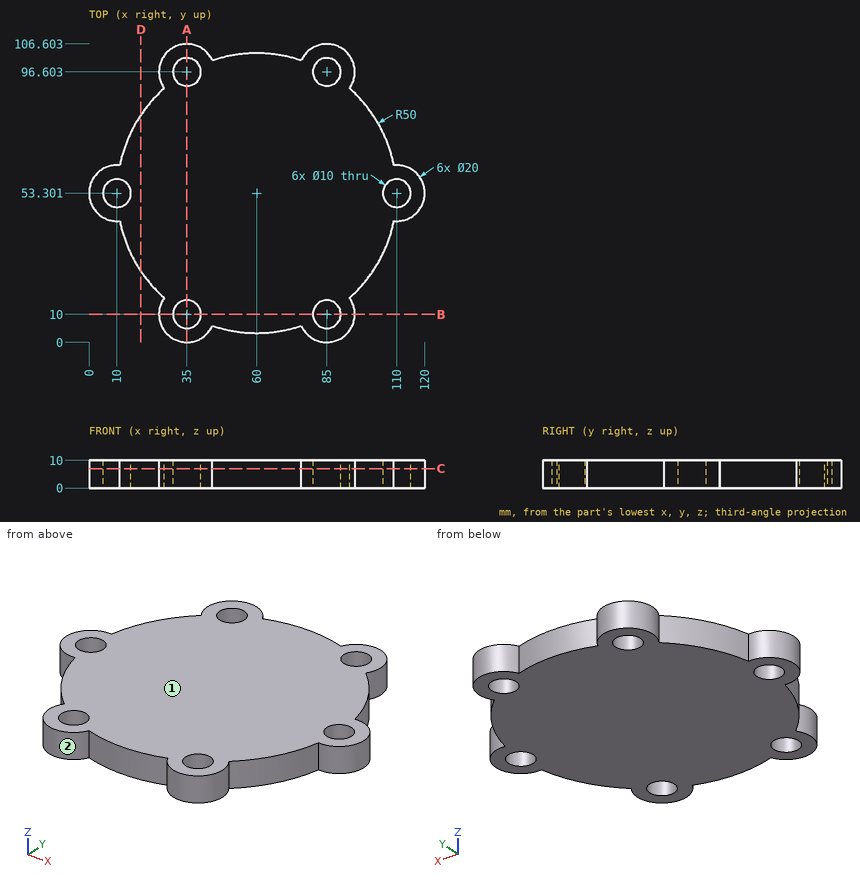
The drawing under review shows one solid part. Ordinate dimensions are in mm from its lowest x, y, z. Give positions to 0.01 mm unless a question says otherwise; leave off trailing zeros. Order: outer loops, then holes, each group sorted by start corner. A loop starts at its lowest first (then second) coordinate and runs counter-clockwise, first axis right, second up. Notation, with made-up numbers: M 17.25,-38.5 L 64.25,-38.5 A21 cw 64.25,-33.5 Z; hole C -3.5,9.25 d5. An arc over 180 degrees is marked long. One line per question, with ' | ' between items. Start each with the question number.
Q1. For pin 1 Ø1.5 at (y, z) = (89, 4) entering from -X; pin 2 Ø6 at (x, z) = (93, 3) entering from +Y, all flat-tipped, find the tip position at first contact; note any pin that passes through.
Q2. We need section B-B (y = 10). Write out the cut boundary in (x, z).
Q3. We need section D-D (x = 18.5). Write out the cut boundary in (y, z).
Q4. For L1, parallel to Y at x = 35, z = 4.5; L2, parallel to Y at x = 10, z = 5.25; L3, parallel to X at y = 9.5, z = 1 (1 decimal), list the stretches that pass through material, from the lowest coordinate up. Write a range as [from, to].
Q5. We need section A-A (x = 35). Write out the cut boundary in (y, z).
Q6. We need section C-C (z = 7). Write out the cut boundary in (x, y).
Q7. The part is to be moulded in two halves that separate along X. For the marked faces 1 and 2, say which applies: +X half, -X half, draft (parallel to the pull), parting line (faces both ways), or undercut.
Returned:
1) pin 1: x = 24.24 | pin 2: y = 105.26
2) outline: M 25,0 L 30,0 L 30,10 L 25,10 Z; M 40,0 L 80,0 L 80,10 L 40,10 Z; M 90,0 L 95,0 L 95,10 L 90,10 Z
3) outline: M 25.41,0 L 81.19,0 L 81.19,10 L 25.41,10 Z
4) L1: [0, 5], [15, 91.6], [101.6, 106.6] | L2: [43.3, 48.3], [58.3, 63.3] | L3: [25, 30], [40, 80], [90, 95]
5) outline: M 0,0 L 5,0 L 5,10 L 0,10 Z; M 15,0 L 91.6,0 L 91.6,10 L 15,10 Z; M 101.6,0 L 106.6,0 L 106.6,10 L 101.6,10 Z
6) outline: M 11,43.35 A50 ccw 26.88,15.84 A10 ccw long 44.12,5.89 A50 ccw 75.88,5.89 A10 ccw long 93.12,15.84 A50 ccw 109,43.35 A10 ccw long 109,63.25 A50 ccw 93.12,90.76 A10 ccw long 75.88,100.71 A50 ccw 44.12,100.71 A10 ccw long 26.88,90.76 A50 ccw 11,63.25 A10 ccw long Z; hole C 10,53.3 d10; hole C 35,10 d10; hole C 35,96.6 d10; hole C 85,10 d10; hole C 85,96.6 d10; hole C 110,53.3 d10
7) face 1: draft | face 2: undercut
